Drawing for the job (mm, zero at the part's lowest x, y, z). A direction names the side the tool comes from. Give positions to 0.01 mm unless a question says otherwise; leave off trailing zeros. Loops run counter-clockwise (first coordinate to the right, second up) from the corner with the lowest first, then second, coordinate; pieces in that order, holes last.
1) Band-saw the part on B-B on z = 13.75. List the corners of the cut face in (x, y), then the cut area to 3 significant figures.
2) Band-saw the part on A-A on x = 40. List the corners of the cut face in (y, z), then the cut area to 3 significant figures.
3) Band-saw the part on C-C on z = 3.75. List the corners of the cut face in (x, y).
4) 3-axis set-ups, long thin cutter, end or side, ignore diameter. For the marked faces 1, 2 and 3: which of +Z, -Z, +X, -X, +Y, -Y reach the whole face in a straight line?
5) Band-saw the part on D-D on x = 14. List the corners of the cut face in (y, z).
6) Wall check: line 1 (X direction, y = 28, z = 13); line 2 (X direction, y = 17.5, z = 1.75); line 3 (Z direction, x = 65, y = 4). Give the ranges that are in metal, low to high.
7) Flat gauge pins, fed straight in: P1, Ø7.5, axis at x = 40, y = 17.5, coming from the +Z side; P2, Ø1.6, axis at x = 77.5, z = 16, coming from the -Y side; P3, Ø5.5, axis at x = 62.5, y = 26.5, coming from the +Z side; P4, Ø2.5, axis at y = 30, z = 17.5, coming from the +X side. Where does each tip first touch, or does it go through?
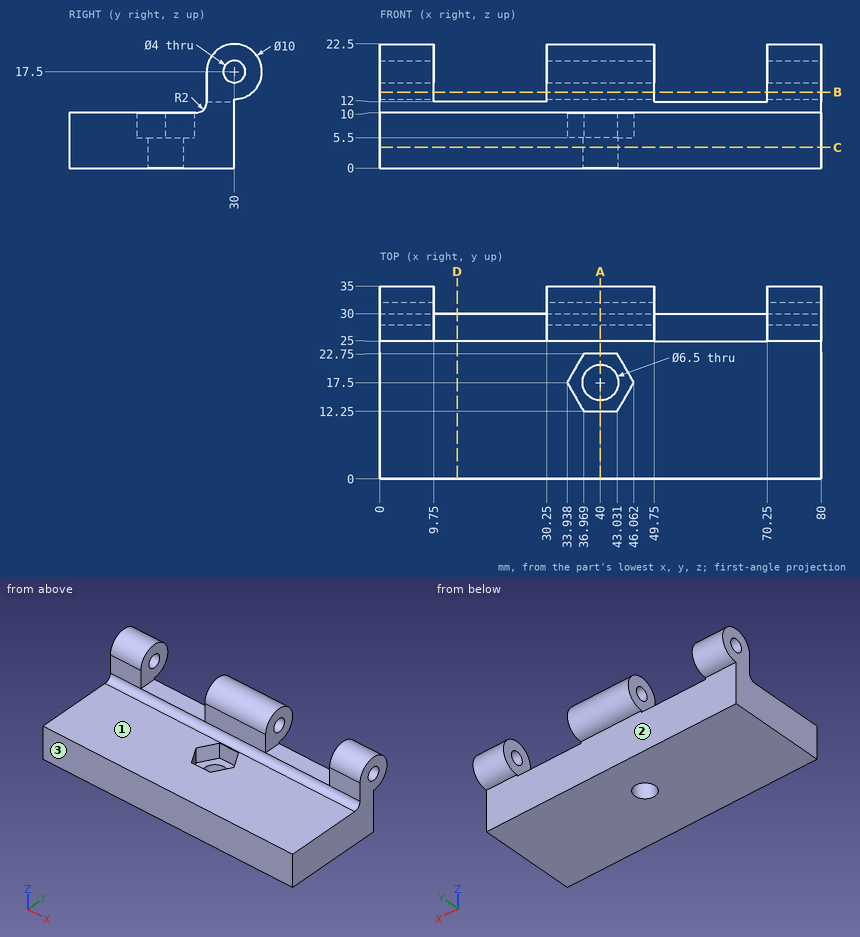
Findings below:
1. outline: (0, 25) - (9.75, 25) - (9.75, 33.31) - (0, 33.31) - close; (30.25, 25) - (49.75, 25) - (49.75, 33.31) - (30.25, 33.31) - close; (70.25, 25) - (80, 25) - (80, 33.31) - (70.25, 33.31) - close
1. area: 324 mm2
2. outline: (0, 0) - (14.25, 0) - (14.25, 5.5) - (12.25, 5.5) - (12.25, 10) - (0, 10) - close; (20.75, 0) - (30, 0) - (30, 12.5) arc R5 ccw (long way) to (25, 17.5) - (25, 12) arc R2 cw to (23, 10) - (22.75, 10) - (22.75, 5.5) - (20.75, 5.5) - close; hole circle Ø4 at (30, 17.5)
2. area: 302 mm2
3. outline: (0, 0) - (80, 0) - (80, 30) - (0, 30) - close; hole circle Ø6.5 at (40, 17.5)
4. face 1: +Z, +X, -X, -Y
4. face 2: -Z, +X, -X, +Y
4. face 3: +Z, -Z, +X, -X, -Y
5. outline: (0, 0) - (30, 0) - (30, 12) - (25, 12) arc R2 cw to (23, 10) - (0, 10) - close
6. line 1: x = 0 to 9.75, 30.25 to 49.75, 70.25 to 80
6. line 2: x = 0 to 36.75, 43.25 to 80
6. line 3: z = 0 to 10
7. P1: stops at z = 5.5
7. P2: stops at y = 25
7. P3: stops at z = 12
7. P4: passes through
